Build history of the part. All positions in model axes, mm. A direction names the side the tool comes from. Round coordinates to 2 decimals unless told otherwise and drop trailing zeros. Order: outer loops, then holes, each group sorted by start corner. A loop starts at its lowest first (then second) coordinate and runs counter-clockwise, first axis right, second up. Notation, with made-up numbers: (-36.5, 64.25) -> (8.5, 64.25) arc R33 ccw to (8.5, 96.25) -> close; hole circle Ø7 at (87, 8.25). An arc over 180 degrees is marked (long way). Answer as a JSON object with one key per item and string values.
from build123d import *

# Parameters (mm, degrees)
SKETCH1_W           = 152.4
SKETCH1_H           = 142.621
BOSS_EXTRUDE1_DEPTH = 3.175
SKETCH2_W           = 3.429
SKETCH2_H           = 32.004
CUT_EXTRUDE1_DEPTH  = 209.750066505
CUT_EXTRUDE2_REACH  = 210.75
SKETCH3_R           = 6.35


with BuildPart() as part:
    # Sketch1 → Boss-Extrude1 (new body)
    with BuildSketch(Plane(origin=(0, 0, 0), x_dir=(1, 0, 0), z_dir=(0, 1, 0))):
        with Locations((76.2, 71.3105)):
            Rectangle(SKETCH1_W, SKETCH1_H)
    extrude(amount=BOSS_EXTRUDE1_DEPTH)

    # Sketch2 → Cut-Extrude1 (cut, through all)
    with BuildSketch(Plane(origin=(0, 3.175, 0), x_dir=(1, 0, 0), z_dir=(0, 1, 0))):
        with Locations((1.7145, 126.619)):
            Rectangle(SKETCH2_W, SKETCH2_H)
        with Locations((150.6855, 126.619)):
            Rectangle(SKETCH2_W, SKETCH2_H)
    extrude(amount=-CUT_EXTRUDE1_DEPTH, mode=Mode.SUBTRACT)

    # Sketch3 → Cut-Extrude2 (cut, up to next)
    with BuildSketch(Plane(origin=(0, 3.175, 0), x_dir=(1, 0, 0), z_dir=(0, 1, 0)), mode=Mode.PRIVATE) as cut_extrude2_sk1:
        with Locations(Location((19.304, 126.746, 0), (0, 0, 270))):
            Circle(SKETCH3_R)
    cut_extrude2_tool1 = extrude(cut_extrude2_sk1.sketch, amount=-CUT_EXTRUDE2_REACH, mode=Mode.PRIVATE) & part.part
    # Sketch3 → Cut-Extrude2 (cut, up to next)
    with BuildSketch(Plane(origin=(0, 3.175, 0), x_dir=(1, 0, 0), z_dir=(0, 1, 0)), mode=Mode.PRIVATE) as cut_extrude2_sk2:
        with Locations(Location((51.054, 126.746, 0), (0, 0, 270))):
            Circle(SKETCH3_R)
    cut_extrude2_tool2 = extrude(cut_extrude2_sk2.sketch, amount=-CUT_EXTRUDE2_REACH, mode=Mode.PRIVATE) & part.part
    # Sketch3 → Cut-Extrude2 (cut, up to next)
    with BuildSketch(Plane(origin=(0, 3.175, 0), x_dir=(1, 0, 0), z_dir=(0, 1, 0)), mode=Mode.PRIVATE) as cut_extrude2_sk3:
        with Locations(Location((82.804, 126.746, 0), (0, 0, 270))):
            Circle(SKETCH3_R)
    cut_extrude2_tool3 = extrude(cut_extrude2_sk3.sketch, amount=-CUT_EXTRUDE2_REACH, mode=Mode.PRIVATE) & part.part
    # Sketch3 → Cut-Extrude2 (cut, up to next)
    with BuildSketch(Plane(origin=(0, 3.175, 0), x_dir=(1, 0, 0), z_dir=(0, 1, 0)), mode=Mode.PRIVATE) as cut_extrude2_sk4:
        with Locations(Location((19.304, 72.644, 0), (0, 0, 270))):
            Circle(SKETCH3_R)
    cut_extrude2_tool4 = extrude(cut_extrude2_sk4.sketch, amount=-CUT_EXTRUDE2_REACH, mode=Mode.PRIVATE) & part.part
    # Sketch3 → Cut-Extrude2 (cut, up to next)
    with BuildSketch(Plane(origin=(0, 3.175, 0), x_dir=(1, 0, 0), z_dir=(0, 1, 0)), mode=Mode.PRIVATE) as cut_extrude2_sk5:
        with Locations(Location((51.054, 72.644, 0), (0, 0, 270))):
            Circle(SKETCH3_R)
    cut_extrude2_tool5 = extrude(cut_extrude2_sk5.sketch, amount=-CUT_EXTRUDE2_REACH, mode=Mode.PRIVATE) & part.part
    # Sketch3 → Cut-Extrude2 (cut, up to next)
    with BuildSketch(Plane(origin=(0, 3.175, 0), x_dir=(1, 0, 0), z_dir=(0, 1, 0)), mode=Mode.PRIVATE) as cut_extrude2_sk6:
        with Locations(Location((82.804, 72.644, 0), (0, 0, 270))):
            Circle(SKETCH3_R)
    cut_extrude2_tool6 = extrude(cut_extrude2_sk6.sketch, amount=-CUT_EXTRUDE2_REACH, mode=Mode.PRIVATE) & part.part
    # Sketch3 → Cut-Extrude2 (cut, up to next)
    with BuildSketch(Plane(origin=(0, 3.175, 0), x_dir=(1, 0, 0), z_dir=(0, 1, 0)), mode=Mode.PRIVATE) as cut_extrude2_sk7:
        with Locations(Location((19.304, 18.542, 0), (0, 0, 270))):
            Circle(SKETCH3_R)
    cut_extrude2_tool7 = extrude(cut_extrude2_sk7.sketch, amount=-CUT_EXTRUDE2_REACH, mode=Mode.PRIVATE) & part.part
    # Sketch3 → Cut-Extrude2 (cut, up to next)
    with BuildSketch(Plane(origin=(0, 3.175, 0), x_dir=(1, 0, 0), z_dir=(0, 1, 0)), mode=Mode.PRIVATE) as cut_extrude2_sk8:
        with Locations(Location((51.054, 18.542, 0), (0, 0, 270))):
            Circle(SKETCH3_R)
    cut_extrude2_tool8 = extrude(cut_extrude2_sk8.sketch, amount=-CUT_EXTRUDE2_REACH, mode=Mode.PRIVATE) & part.part
    # Sketch3 → Cut-Extrude2 (cut, up to next)
    with BuildSketch(Plane(origin=(0, 3.175, 0), x_dir=(1, 0, 0), z_dir=(0, 1, 0)), mode=Mode.PRIVATE) as cut_extrude2_sk9:
        with Locations(Location((82.804, 18.542, 0), (0, 0, 270))):
            Circle(SKETCH3_R)
    cut_extrude2_tool9 = extrude(cut_extrude2_sk9.sketch, amount=-CUT_EXTRUDE2_REACH, mode=Mode.PRIVATE) & part.part
    # Sketch3 → Cut-Extrude2 (cut, up to next)
    with BuildSketch(Plane(origin=(0, 3.175, 0), x_dir=(1, 0, 0), z_dir=(0, 1, 0)), mode=Mode.PRIVATE) as cut_extrude2_sk10:
        with BuildLine():
            Line((22.479, 107.696), (22.479, 91.821))
            ThreePointArc((22.479, 91.821), (19.304, 88.646), (16.129, 91.821))
            Line((16.129, 91.821), (16.129, 107.696))
            ThreePointArc((16.129, 107.696), (19.304, 110.871), (22.479, 107.696))
        make_face()
    cut_extrude2_tool10 = extrude(cut_extrude2_sk10.sketch, amount=-CUT_EXTRUDE2_REACH, mode=Mode.PRIVATE) & part.part
    # Sketch3 → Cut-Extrude2 (cut, up to next)
    with BuildSketch(Plane(origin=(0, 3.175, 0), x_dir=(1, 0, 0), z_dir=(0, 1, 0)), mode=Mode.PRIVATE) as cut_extrude2_sk11:
        with BuildLine():
            Line((54.229, 107.696), (54.229, 91.821))
            ThreePointArc((54.229, 91.821), (51.054, 88.646), (47.879, 91.821))
            Line((47.879, 91.821), (47.879, 107.696))
            ThreePointArc((47.879, 107.696), (51.054, 110.871), (54.229, 107.696))
        make_face()
    cut_extrude2_tool11 = extrude(cut_extrude2_sk11.sketch, amount=-CUT_EXTRUDE2_REACH, mode=Mode.PRIVATE) & part.part
    # Sketch3 → Cut-Extrude2 (cut, up to next)
    with BuildSketch(Plane(origin=(0, 3.175, 0), x_dir=(1, 0, 0), z_dir=(0, 1, 0)), mode=Mode.PRIVATE) as cut_extrude2_sk12:
        with BuildLine():
            Line((85.979, 107.696), (85.979, 91.821))
            ThreePointArc((85.979, 91.821), (82.804, 88.646), (79.629, 91.821))
            Line((79.629, 91.821), (79.629, 107.696))
            ThreePointArc((79.629, 107.696), (82.804, 110.871), (85.979, 107.696))
        make_face()
    cut_extrude2_tool12 = extrude(cut_extrude2_sk12.sketch, amount=-CUT_EXTRUDE2_REACH, mode=Mode.PRIVATE) & part.part
    # Sketch3 → Cut-Extrude2 (cut, up to next)
    with BuildSketch(Plane(origin=(0, 3.175, 0), x_dir=(1, 0, 0), z_dir=(0, 1, 0)), mode=Mode.PRIVATE) as cut_extrude2_sk13:
        with BuildLine():
            Line((22.479, 53.594), (22.479, 37.719))
            ThreePointArc((22.479, 37.719), (19.304, 34.544), (16.129, 37.719))
            Line((16.129, 37.719), (16.129, 53.594))
            ThreePointArc((16.129, 53.594), (19.304, 56.769), (22.479, 53.594))
        make_face()
    cut_extrude2_tool13 = extrude(cut_extrude2_sk13.sketch, amount=-CUT_EXTRUDE2_REACH, mode=Mode.PRIVATE) & part.part
    # Sketch3 → Cut-Extrude2 (cut, up to next)
    with BuildSketch(Plane(origin=(0, 3.175, 0), x_dir=(1, 0, 0), z_dir=(0, 1, 0)), mode=Mode.PRIVATE) as cut_extrude2_sk14:
        with BuildLine():
            Line((54.229, 53.594), (54.229, 37.719))
            ThreePointArc((54.229, 37.719), (51.054, 34.544), (47.879, 37.719))
            Line((47.879, 37.719), (47.879, 53.594))
            ThreePointArc((47.879, 53.594), (51.054, 56.769), (54.229, 53.594))
        make_face()
    cut_extrude2_tool14 = extrude(cut_extrude2_sk14.sketch, amount=-CUT_EXTRUDE2_REACH, mode=Mode.PRIVATE) & part.part
    # Sketch3 → Cut-Extrude2 (cut, up to next)
    with BuildSketch(Plane(origin=(0, 3.175, 0), x_dir=(1, 0, 0), z_dir=(0, 1, 0)), mode=Mode.PRIVATE) as cut_extrude2_sk15:
        with BuildLine():
            Line((85.979, 53.594), (85.979, 37.719))
            ThreePointArc((85.979, 37.719), (82.804, 34.544), (79.629, 37.719))
            Line((79.629, 37.719), (79.629, 53.594))
            ThreePointArc((79.629, 53.594), (82.804, 56.769), (85.979, 53.594))
        make_face()
    cut_extrude2_tool15 = extrude(cut_extrude2_sk15.sketch, amount=-CUT_EXTRUDE2_REACH, mode=Mode.PRIVATE) & part.part
    add(cut_extrude2_tool1.solids().sort_by_distance((19.304, 3.175, -126.746))[0], mode=Mode.SUBTRACT)
    add(cut_extrude2_tool2.solids().sort_by_distance((51.054, 3.175, -126.746))[0], mode=Mode.SUBTRACT)
    add(cut_extrude2_tool3.solids().sort_by_distance((82.804, 3.175, -126.746))[0], mode=Mode.SUBTRACT)
    add(cut_extrude2_tool4.solids().sort_by_distance((19.304, 3.175, -72.644))[0], mode=Mode.SUBTRACT)
    add(cut_extrude2_tool5.solids().sort_by_distance((51.054, 3.175, -72.644))[0], mode=Mode.SUBTRACT)
    add(cut_extrude2_tool6.solids().sort_by_distance((82.804, 3.175, -72.644))[0], mode=Mode.SUBTRACT)
    add(cut_extrude2_tool7.solids().sort_by_distance((19.304, 3.175, -18.542))[0], mode=Mode.SUBTRACT)
    add(cut_extrude2_tool8.solids().sort_by_distance((51.054, 3.175, -18.542))[0], mode=Mode.SUBTRACT)
    add(cut_extrude2_tool9.solids().sort_by_distance((82.804, 3.175, -18.542))[0], mode=Mode.SUBTRACT)
    add(cut_extrude2_tool10.solids().sort_by_distance((19.304, 3.175, -99.7585))[0], mode=Mode.SUBTRACT)
    add(cut_extrude2_tool11.solids().sort_by_distance((51.054, 3.175, -99.7585))[0], mode=Mode.SUBTRACT)
    add(cut_extrude2_tool12.solids().sort_by_distance((82.804, 3.175, -99.7585))[0], mode=Mode.SUBTRACT)
    add(cut_extrude2_tool13.solids().sort_by_distance((19.304, 3.175, -45.6565))[0], mode=Mode.SUBTRACT)
    add(cut_extrude2_tool14.solids().sort_by_distance((51.054, 3.175, -45.6565))[0], mode=Mode.SUBTRACT)
    add(cut_extrude2_tool15.solids().sort_by_distance((82.804, 3.175, -45.6565))[0], mode=Mode.SUBTRACT)


solid = part.part
1) Which spindle directions (+Z, -Z, +X, -X, +Y, -Y) get a long thin tool onto all of the face, cutting with end or side? Do faces 1 (the face through (2, 2, -110.617)), 2 (the face through (75, 2, -142.621)), 3 (the face through (85.979, 2, -100)). Say none if no direction does.
Checked values:
{"face 1": "-Z, -X, +Y, -Y", "face 2": "-Z, +X, -X, +Y, -Y", "face 3": "+Y, -Y"}
2) Flat gauge pins, fed straight in: pin 1 Ø1.6 at (x, y) = (2.5, 1.5) entering from -Z; pin 2 Ø1 at (y, z) = (1, -40) entering from -X; pin 3 Ø7.5 at (x, z) = (82.804, -72.644) entering from -Y; pin 4 Ø1.5 at (y, z) = (1.5, -118.5) entering from -X. Where does each tip first touch, or does it go through?
Checked values:
{"pin 1": "stops at z = -110.62", "pin 2": "stops at x = 0", "pin 3": "passes through", "pin 4": "stops at x = 3.43"}
3) Cut at B-B, the plane y = 0.85. Count the separate pieces of the cut face and the enclosed holes in it, plus the area to 3 significant figures.
Checked values:
{"separate pieces": "1", "enclosed holes": "15", "area": "19,600 mm²"}
4) Cut at C-C, the plane z = -70. Give the cut face in (x, y) (3 decimals), plus the area to 3 significant figures.
Checked values:
{"outline": "(0, 0) -> (13.531, 0) -> (13.531, 3.175) -> (0, 3.175) -> close; (25.077, 0) -> (45.281, 0) -> (45.281, 3.175) -> (25.077, 3.175) -> close; (56.827, 0) -> (77.031, 0) -> (77.031, 3.175) -> (56.827, 3.175) -> close; (88.577, 0) -> (152.4, 0) -> (152.4, 3.175) -> (88.577, 3.175) -> close", "area": "374 mm²"}
5) Cut at A-A, the plane z = -51.5. Give the cut face in (x, y) (3 decimals).
Checked values:
{"outline": "(0, 0) -> (16.129, 0) -> (16.129, 3.175) -> (0, 3.175) -> close; (22.479, 0) -> (47.879, 0) -> (47.879, 3.175) -> (22.479, 3.175) -> close; (54.229, 0) -> (79.629, 0) -> (79.629, 3.175) -> (54.229, 3.175) -> close; (85.979, 0) -> (152.4, 0) -> (152.4, 3.175) -> (85.979, 3.175) -> close"}
6) Pull direction X, two halves, no side cores. Call faces 4 (the face through (19.374, 1.61, -34.545)), 5 (the face through (151, 2, -110.617)), 6 (the face through (3.429, 2, -126)): pulls with the +X half, pulls with the -X half, needs draft (parallel to the pull), parting line crosses it, or undercut.
Checked values:
{"face 4": "undercut", "face 5": "needs draft", "face 6": "pulls with the -X half"}
7) Probe L1, parallel to X at y = 0.5, z = -43.5; L2, parallel to Z at x = 19.5, y = 2.55; L3, parallel to X at y = 2.8, z = -72.5. List the from-to ranges inside material, lowest first. Write a range as from..to.
Checked values:
{"L1": "x = 0..16.13, 22.48..47.88, 54.23..79.63, 85.98..152.4", "L2": "z = -142.62..-133.09, -120.4..-110.86, -88.65..-78.99, -66.3..-56.76, -34.55..-24.89, -12.2..0", "L3": "x = 0..12.96, 25.65..44.71, 57.4..76.46, 89.15..152.4"}
